from build123d import *

# Parameters (mm, degrees)
SKETCH2_R           = 17.25
SKETCH2_R_2         = 15
BOSS_EXTRUDE4_DEPTH = 20
SKETCH4_R           = 20
SKETCH4_R_2         = 15
BOSS_EXTRUDE6_DEPTH = 10
BOSS_EXTRUDE7_START = 10
SKETCH5_R           = 15
SKETCH5_R_2         = 12.5
BOSS_EXTRUDE7_DEPTH = 10


with BuildPart() as part:
    # Sketch2 → Boss-Extrude4 (new body)
    with BuildSketch(Plane(origin=(0, 0, 0), x_dir=(1, 0, 0), z_dir=(0, 1, 0))):
        Circle(SKETCH2_R)
        Circle(SKETCH2_R_2, mode=Mode.SUBTRACT)
    extrude(amount=BOSS_EXTRUDE4_DEPTH)

    # Sketch4 → Boss-Extrude6 (add)
    with BuildSketch(Plane(origin=(0, 0, 0), x_dir=(1, 0, 0), z_dir=(0, 1, 0))):
        Circle(SKETCH4_R)
        Circle(SKETCH4_R_2, mode=Mode.SUBTRACT)
    extrude(amount=BOSS_EXTRUDE6_DEPTH)

    # Sketch5 → Boss-Extrude7 (add)
    with BuildSketch(Plane(origin=(0, 0, 0), x_dir=(1, 0, 0), z_dir=(0, 1, 0)).offset(BOSS_EXTRUDE7_START)):
        Circle(SKETCH5_R)
        Circle(SKETCH5_R_2, mode=Mode.SUBTRACT)
    extrude(amount=BOSS_EXTRUDE7_DEPTH)


solid = part.part
Model file for the job. Use its own axes, mm. A direction names the side the tool comes from. Coordinates: 2 decimals unless noted, no trailing zeros. Order: outer loops, then holes, each group sorted by start corner. A loop starts at its lowest first (then second) coordinate and runs counter-clockwise, first axis right, second up. Notation, with made-up numbers: M 26,-7.75 L 83,-7.75 A12 ccw 83,5.25 Z; hole C -25.5,2.25 d11. An arc over 180 degrees is marked long. Return JSON: item names as keys, results as strings.
1. Saw through at D-D (z = -14.5). Give the cut face in (x, y).
Ans:
{"outline": "M -13.77,0 L -3.84,0 L -3.84,10 L 3.84,10 L 3.84,0 L 13.77,0 L 13.77,10 L 9.34,10 L 9.34,20 L -9.34,20 L -9.34,10 L -13.77,10 Z"}
2. Saw through at B-B (x = 0). Give the cut face in (y, z).
Ans:
{"outline": "M 0,-20 L 10,-20 L 10,-17.25 L 20,-17.25 L 20,-12.5 L 10,-12.5 L 10,-15 L 0,-15 Z; M 0,15 L 10,15 L 10,12.5 L 20,12.5 L 20,17.25 L 10,17.25 L 10,20 L 0,20 Z"}
3. Saw through at A-A (z = 0). Give the cut face in (x, y).
Ans:
{"outline": "M -20,0 L -15,0 L -15,10 L -12.5,10 L -12.5,20 L -17.25,20 L -17.25,10 L -20,10 Z; M 12.5,10 L 15,10 L 15,0 L 20,0 L 20,10 L 17.25,10 L 17.25,20 L 12.5,20 Z"}
4. Drill centre lines: probe 1 along X at (y, z) = (15.25, 0); probe 2 along Z at (x, y) = (0, 6.5). Where is each one in solid material? Low to high.
Ans:
{"probe 1": "-17.25 to -12.5, 12.5 to 17.25", "probe 2": "-20 to -15, 15 to 20"}
5. Tool access for faces 1 (the face through (-15, 10, 9)), 2 (the face through (11.923, 14.93, -3.755)), 3 (the face through (-14.985, 4.93, -0.66)): list every direction of +Z, -Z, +X, -X, +Y, -Y with a clear straight run to the whole face (end or side of a thin tool).
Ans:
{"face 1": "+Y", "face 2": "+Y, -Y", "face 3": "-Y"}
6. Saw through at C-C (y = 15.5). Give the cut face in (x, z).
Ans:
{"outline": "C 0,0 d34.5; hole C 0,0 d25"}
7. Flat gauge pins, fed straight in: pin 1 (24 mm diameter, centred on x = 0, z = 0, fed in from +Y); pin 2 (12 mm diameter, centred on y = 17.5, z = 14, fed in from +X); pin 3 (2 mm diameter, centred on x = 15.5, z = 1, fed in from -Y); pin 4 (2 mm diameter, centred on x = -4, y = 14, fed in from -Z). Where does each tip first touch, or does it go through?
Ans:
{"pin 1": "through", "pin 2": "x = 15.28", "pin 3": "y = 0", "pin 4": "z = -16.99"}
8. Pull direction X, two halves, no side cores. Call faces 4 (the face through (-3.4, 10, -12.3)), 5 (the face through (3, 0, -15)), 6 (the face through (16.453, 14.93, -5.181)): +X half, -X half, draft (parallel to the pull), parting line (faces both ways), or undercut.
Ans:
{"face 4": "undercut", "face 5": "draft", "face 6": "parting line"}
